from build123d import *

# Parameters (mm, degrees)
F1_DEPTH = 3.175


# Not quite as in the source:
# - a length typed as a fraction of an inch, garbled in the dataset ("3 / 203.2 mm" for 3/8 in), is restored
# - a feature names something its author has since deleted; it is built from what else it names


with BuildPart() as f1:
    # F0 (on Top) → F1 (new body)
    with BuildSketch(Plane.XY):
        with BuildLine():
            Line((22.4136457592, 16), (0, 16))
            Line((0, 16), (-22.4136457592, 16))
            ThreePointArc((-22.4136457592, 16), (-25.9491796652, 14.5355339059), (-27.4136457592, 11))
            Line((-27.4136457592, 11), (-27.4136457592, -15.5))
            ThreePointArc((-27.4136457592, -15.5), (-25.9491796652, -19.0355339059), (-22.4136457592, -20.5))
            Line((-22.4136457592, -20.5), (-6.0621778265, -20.5))
            ThreePointArc((-6.0621778265, -20.5), (-1.8117333157, -10.238519216), (7, -17))
            ThreePointArc((7, -17), (6.761480784, -18.8117333157), (6.0621778265, -20.5))
            Line((6.0621778265, -20.5), (22.4136457592, -20.5))
            ThreePointArc((22.4136457592, -20.5), (25.9491796652, -19.0355339059), (27.4136457592, -15.5))
            Line((27.4136457592, -15.5), (27.4136457592, 11))
            ThreePointArc((27.4136457592, 11), (25.9491796652, 14.5355339059), (22.4136457592, 16))
        make_face()
        Polygon((22, 9), (22, -9), (-22, -9), (-22, 9), (0, 9), align=None, mode=Mode.SUBTRACT)
        with BuildLine():
            ThreePointArc((1.5875, 12.3080683509), (1.1225320151, 11.1855363358), (0, 10.7205683509))
            ThreePointArc((0, 10.7205683509), (-1.5875, 12.3080683509), (0, 13.8955683509))
            ThreePointArc((0, 13.8955683509), (1.1225320151, 13.4306003661), (1.5875, 12.3080683509))
        make_face(mode=Mode.SUBTRACT)
        Polygon((-22, -9), (22, -9), (22, 9), (0, 9), (-22, 9), align=None)
        with BuildLine():
            Line((-18.4078, 6.75), (0, 6.75))
            Line((0, 6.75), (18.4078, 6.75))
            ThreePointArc((18.4078, 6.75), (19.5, 7.8422), (20.5922, 6.75))
            ThreePointArc((20.5922, 6.75), (20.2723020264, 5.9776979736), (19.5, 5.6578))
            Line((19.5, 5.6578), (19.5, -5.6578))
            ThreePointArc((19.5, -5.6578), (20.2723020264, -5.9776979736), (20.5922, -6.75))
            ThreePointArc((20.5922, -6.75), (19.5, -7.8422), (18.4078, -6.75))
            Line((18.4078, -6.75), (-18.4078, -6.75))
            ThreePointArc((-18.4078, -6.75), (-20.2723020264, -7.5223020264), (-19.5, -5.6578))
            Line((-19.5, -5.6578), (-19.5, 5.6578))
            ThreePointArc((-19.5, 5.6578), (-20.2723020264, 7.5223020264), (-18.4078, 6.75))
        make_face(mode=Mode.SUBTRACT)
        with BuildLine():
            Line((18.4078, 6.75), (0, 6.75))
            Line((0, 6.75), (-18.4078, 6.75))
            ThreePointArc((-18.4078, 6.75), (-18.7276979736, 5.9776979736), (-19.5, 5.6578))
            Line((-19.5, 5.6578), (-19.5, -5.6578))
            ThreePointArc((-19.5, -5.6578), (-18.7276979736, -5.9776979736), (-18.4078, -6.75))
            Line((-18.4078, -6.75), (18.4078, -6.75))
            ThreePointArc((18.4078, -6.75), (18.7276979736, -5.9776979736), (19.5, -5.6578))
            Line((19.5, -5.6578), (19.5, 5.6578))
            ThreePointArc((19.5, 5.6578), (18.7276979736, 5.9776979736), (18.4078, 6.75))
        make_face()
        with BuildLine():
            ThreePointArc((7, -17), (-1.8117333157, -10.238519216), (-6.0621778265, -20.5))
            Line((-6.0621778265, -20.5), (2.55e-08, -20.5))
            Line((2.55e-08, -20.5), (6.0621778265, -20.5))
            ThreePointArc((6.0621778265, -20.5), (6.761480784, -18.8117333157), (7, -17))
        make_face()
        with BuildLine():
            ThreePointArc((3.5, -17), (2.4748737432, -19.4748737251), (2.55e-08, -20.5))
            ThreePointArc((2.55e-08, -20.5), (-2.4748737432, -14.5251262749), (3.5, -17))
        make_face(mode=Mode.SUBTRACT)
        with BuildLine():
            Line((2.55e-08, -20.5), (-6.0621778265, -20.5))
            ThreePointArc((-6.0621778265, -20.5), (0, -24), (6.0621778265, -20.5))
            Line((6.0621778265, -20.5), (2.55e-08, -20.5))
        make_face()
    extrude(amount=F1_DEPTH)


solid = f1.part
Design review of the part built by this model. Coordinates are the model's own, in mm. A direction names the side the tool comes from. Give positions to 0.01 mm unless a question says otherwise; leave off trailing zeros. Write each loop counter-clockwise with the first axis right and the second up, starting at its lowest first coordinate (ties: lowest second). Pieces come first, ordered by that corner, then holes. Notation, with made-up numbers: M 52,45 L 86,45 A26 ccw 86,66 Z; hole C 3.5,85.5 d2. An arc over 180 degrees is marked long. Answer as a JSON object with one key per item and string values. Group by question number.
1) We need section B-B (x = 16). Give the boundary of the cut face in (y, z) (3 decimals).
2) Tool access review of faces 1 (the face through (14, -20.5, 2)), 2 (the face through (-14, -20.5, 2)), 3 (the face through (0, 16, 2)): name each direction out of +Z, -Z, +X, -X, +Y, -Y from which nothing blocks a thin tool from reaching the whole face with its end or side.
3) For line 1 along Y through (x, z) = (-19.5, 1.6); line 2 along X through (y, z) = (6.75, 1.3); line 3 along X through (y, z) = (-6, 1.3), list the stretches that pass through material, from the lowest coordinate up.
4) We need section A-A (z = 0.75). Count the separate pieces of the cut face and the enclosed holes in it, and give its area (3 significant figures).
5) We need section C-C (x = 4.5). Give the boundary of the cut face in (y, z) (3 decimals), and give its area (3 significant figures).
Answer key:
{
 "1": {"outline": "M -20.5,0 L 16,0 L 16,3.175 L -20.5,3.175 Z"},
 "2": {"face 1": "+Z, -Z, +X, -Y", "face 2": "+Z, -Z, -X, -Y", "face 3": "+Z, -Z, +X, -X, +Y"},
 "3": {"line 1": "y = -20.5 to -7.84, -5.66 to 5.66, 7.84 to 16", "line 2": "x = -27.41 to -20.59, -18.41 to 18.41, 20.59 to 27.41", "line 3": "x = -27.41 to -20.29, -18.71 to 18.71, 20.29 to 27.41"},
 "4": {"separate pieces": "1", "enclosed holes": "6", "area": "1,950 mm²"},
 "5": {"outline": "M -22.362,0 L 16,0 L 16,3.175 L -22.362,3.175 Z", "area": "122 mm²"}
}
